```python
from build123d import *

# Parameters (mm, degrees)
SKETCH3_R           = 63.5
SKETCH3_R_2         = 57.15
BOSS_EXTRUDE1_DEPTH = 19.05


with BuildPart() as part:
    # Sketch2 → Revolve1 (revolve)
    with BuildSketch(Plane.XY):
        Polygon((-45.72, 0), (-52.07, 0), (-65.405, 12.7), (-57.15, 12.7), align=None)
    revolve(axis=Axis((0, 0, 0), (0, 1, 0)))

    # Sketch3 → Boss-Extrude1 (add)
    with BuildSketch(Plane(origin=(0, 12.7, 0), x_dir=(1, 0, 0), z_dir=(0, 1, 0))):
        Circle(SKETCH3_R)
        Circle(SKETCH3_R_2, mode=Mode.SUBTRACT)
    extrude(amount=BOSS_EXTRUDE1_DEPTH)


solid = part.part
```
The listing builds one solid part. Answer for the finished solid, in the listing's coordinates (mm). A direction names the side the tool comes from. Round coordinates to 2 decimals unless told otherwise and drop trailing zeros. Loops run counter-clockwise (first coordinate to the right, second up) from the corner with the lowest first, then second, coordinate; pieces in that order, holes last.
Q1. Section B-B, the plane z = 0 is taken. Determine the outline of the cut face in (x, y) (3 decimals).
Q2. Which of the six approach directions +Z, -Z, +X, -X, +Y, -Y give full straight-line access (tool end or side, diameter ignored) to faces 4 (the face through (54, 12.7, 34)), 5 (the face through (0, 0, -46))?
Q3. Find the intervals of material crossed by line 1 (Z direction, x = 0, y = 20); line 2 (X direction, y = 29.5, z = -11.5), in increasing order.
Q4. Given pin 1 Ø5 at (y, z) = (22.5, 2.5) entering from +X; pin 2 Ø1 at (y, z) = (22, 14.5) entering from +X; pin 3 Ø6 at (x, z) = (-44.5, 17) entering from -Y; pin 4 Ø6 at (y, z) = (16.5, -8) entering from -X, each flat-ended and moving along its own axis, determine where each tip first touches the part or whether it passes through.
Q5. Section C-C, the plane y = 25 is taken. Determine the outline of the cut face in (x, z).
Q6. Section D-D, the plane y = 3.5 is taken. Determine the outline of the cut face in (x, z) (3 decimals), then the cut area to 3 significant figures.
Q7. For a pull along Z with two mould halves and no side action, classify faces 1 (the face through (-57, 31.75, -10)), 2 (the face through (6.89, 0.79, 52.45)), 3 (the face through (-42.75, 0.62, -17.72)) as released by +Z, released by -Z, zero draft, split by the parting line, or undercut.
Q8. Section A-A, the plane x = 0 is taken. Determine the outline of the cut face in (y, z) (3 decimals), then the cut area to 3 significant figures.
Completed:
1. outline: (-65.405, 12.7) - (-52.07, 0) - (-45.72, 0) - (-57.15, 12.7) - (-57.15, 31.75) - (-63.5, 31.75) - (-63.5, 12.7) - close; (45.72, 0) - (52.07, 0) - (65.405, 12.7) - (63.5, 12.7) - (63.5, 31.75) - (57.15, 31.75) - (57.15, 12.7) - close
2. face 4: +Y
2. face 5: +Z, -Z, +X, -X, -Y
3. line 1: z = -63.5 to -57.15, 57.15 to 63.5
3. line 2: x = -62.45 to -55.98, 55.98 to 62.45
4. pin 1: stops at x = 63.5
4. pin 2: stops at x = 61.94
4. pin 3: stops at y = 0
4. pin 4: stops at x = -63.3
5. outline: circle Ø127 at (0, 0); hole circle Ø114.3 at (0, 0)
6. outline: circle Ø111.49 at (0, 0); hole circle Ø97.74 at (0, 0)
6. area: 2,260 mm2
7. face 1: zero draft
7. face 2: split by the parting line
7. face 3: undercut
8. outline: (0, -52.07) - (12.7, -65.405) - (12.7, -63.5) - (31.75, -63.5) - (31.75, -57.15) - (12.7, -57.15) - (0, -45.72) - close; (0, 45.72) - (12.7, 57.15) - (31.75, 57.15) - (31.75, 63.5) - (12.7, 63.5) - (12.7, 65.405) - (0, 52.07) - close
8. area: 427 mm2
